The figure shows three views and two pictorial views of one solid part (mm, origin at its lowest corner). Answer the questions. Round coordinates to 2 decimals unless told otherwise and drop trailing zeros. Order: outer loops, then holes, each group sorted by start corner. A loop starts at its lowest first (then second) coordinate and runs counter-clockwise, first axis right, second up. Notation, with made-up numbers: (29, 55.5) -> (42, 55.5) arc R26 cw to (42, 76.5) -> close; hole circle Ø2 at (80.5, -28.5). An arc over 180 degrees is marked (long way). Answer as a JSON object with one key per item and string values. Group by question number.
Item 1: Given P1, Ø1, axis at y = 1.5, z = 8.5, coming from the -X side (1 decimal); P2, Ø4, axis at x = 7, y = 8.5, coming from the +Z side; P3, Ø1.5, axis at x = 5, y = 2.5, coming from the -Z side; P4, Ø3, axis at y = 5, z = 5, coming from the -X side, each flat-ended and moving along its own axis, determine where each tip first touches the part or whether it passes through.
Item 2: Section C-C, the plane x = 2.25 is taken. Write down the section's boundary in (y, z).
Item 3: Section D-D, the plane x = 8 is taken. Write down the section's boundary in (y, z) (1 decimal), plus the area to 3 significant figures.
Item 4: Consider probe 1 along Z at (x, y) = (5.75, 5); probe 2 along Z at (x, y) = (4.25, 4.25) (1 decimal); probe 3 along Y at (x, z) = (2.5, 7) (1 decimal). Determine where each line is inside the solid, lowest interval first. Write a range as from..to.
Item 5: Section A-A, the plane y = 5 is taken. Write down the section's boundary in (x, z) (1 decimal).
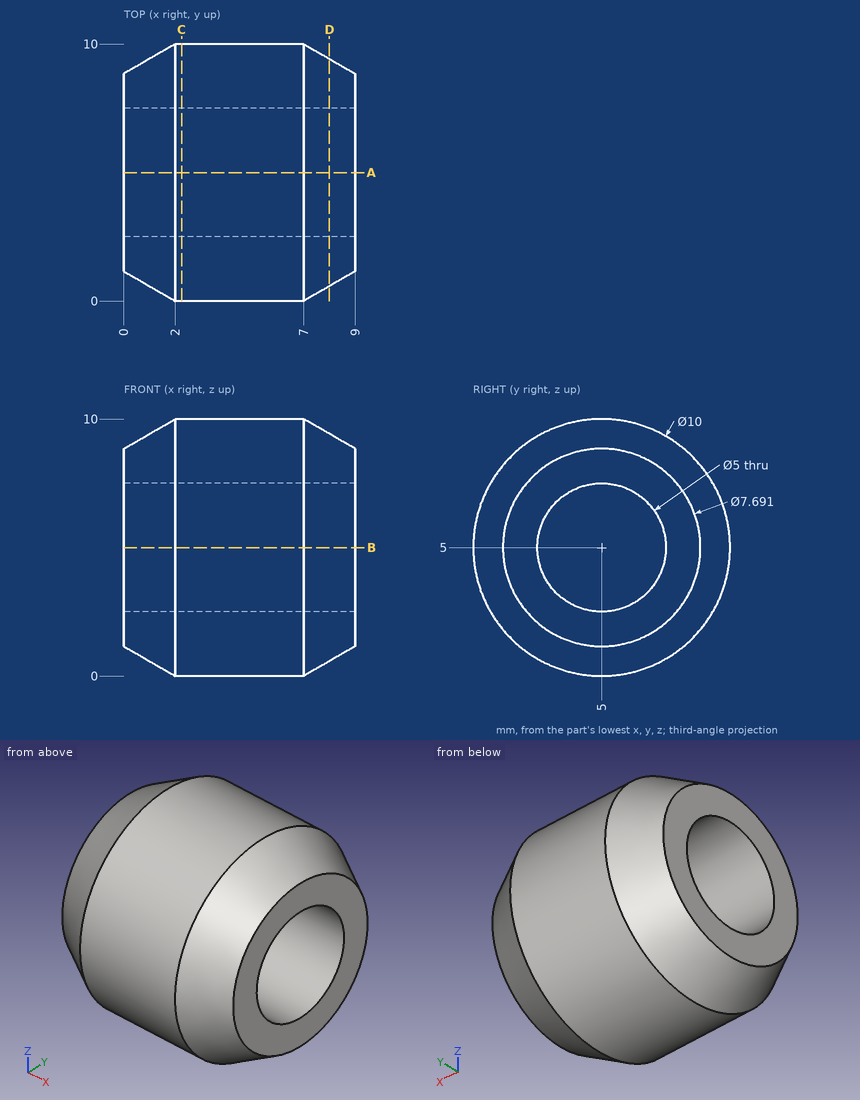
Values found:
{
 "1": {"P1": "x = 1", "P2": "z = 9.77", "P3": "z = 0.32", "P4": "through"},
 "2": {"outline": "circle Ø10 at (5, 5); hole circle Ø5 at (5, 5)"},
 "3": {"outline": "circle Ø8.8 at (5, 5); hole circle Ø5 at (5, 5)", "area": "41.8 mm2"},
 "4": {"probe 1": "0..2.5, 7.5..10", "probe 2": "0.1..2.6, 7.4..9.9", "probe 3": "0.4..3.5, 6.5..9.6"},
 "5": {"outline": "(0, 1.2) -> (2, 0) -> (7, 0) -> (9, 1.2) -> (9, 2.5) -> (0, 2.5) -> close; (0, 7.5) -> (9, 7.5) -> (9, 8.8) -> (7, 10) -> (2, 10) -> (0, 8.8) -> close"}
}
